Autodesk Inventor part; units mm, degrees
ref_plane "YZ Plane" through (0, 0, 0) normal (1, 0, 0) x (0, 1, 0)
ref_plane "XZ Plane" through (0, 0, 0) normal (0, 1, 0) x (-1, 0, 0)
ref_plane "XY Plane" through (0, 0, 0) normal (0, 0, 1) x (1, 0, 0)
sketch "Sketch11" plane through (0, 0, 0) normal (0, 1, 0) x (-1, 0, 0)
  circle A0 centre (0, 0) radius 26
  circle A1 centre (0, 0) radius 24
  circle A2 centre (0, 0) radius 31
  circle A3 centre (0, 0) radius 55
  line L0 (35.5726, 38.3198) -> (39.3254, 31.8198)
  line L1 (39.3254, 31.8198) -> (35.5726, 25.3198)
  line L2 (35.5726, 25.3198) -> (28.067, 25.3198)
  line L3 (28.067, 25.3198) -> (24.3143, 31.8198)
  line L4 (24.3143, 31.8198) -> (28.067, 38.3198)
  line L5 (28.067, 38.3198) -> (35.5726, 38.3198)
  line L6 (0, 0) -> (31.8198, 31.8198) construction
  line L7 (0, 0) -> (45, 0) construction
  line L8 (35.5726, 38.3198) -> (28.067, 25.3198) construction
  line L9 (28.067, 38.3198) -> (35.5726, 25.3198) construction
  line L10 (39.3254, 31.8198) -> (24.3143, 31.8198) construction
  line L11 (0, 52.6213) -> (0, 85)
  line L12 (0, 85) -> (-16, 85)
  line L13 (-16, 85) -> (-16, 52.6213)
  line L14 (0, 64) -> (0, 58.5)
  line L15 (-16, 52.6213) -> (0, 52.6213)
  line L16 (0, 52.6213) -> (-16, 52.6213)
  line L17 (-16, 52.6213) -> (-16, 44.6213)
  line L18 (-16, 44.6213) -> (0, 44.6213)
  line L19 (0, 44.6213) -> (0, 52.6213)
  line L20 (0, 68.8106) -> (-43, 68.8106)
  line L21 (-43, 68.8106) -> (-43, 250.8106)
  line L22 (-43, 250.8106) -> (0, 250.8106)
  line L23 (0, 250.8106) -> (0, 68.8106)
  dimension "oOuterDia" = 110
  dimension "oPipeDia" = 52
  dimension "oPipeWall" = 2
  dimension "oPipeLenght" = 5
  dimension "oKdia" = 45
  dimension "d70" = 45
  dimension "oSW" = 13
  dimension "oCenterTop" = 85
  dimension "d78" = 16
  dimension "d86" = 8
  dimension "oActuatorDia" = 43
  dimension "oActuatorLenght" = 182
extrude "Extrusion12" add sketch "Sketch11" along normal mid plane 52 contours A0
extrude "Extrusion13" add sketch "Sketch11" along normal mid plane 42 contours A2
extrude "Extrusion14" add sketch "Sketch11" along normal mid plane 22 contours L17 L18 L19 L11 A3 | A3 L11 L15 | L15 L19 L18 L17 | L0 L1 L2 L3 L4 L5
extrude "Extrusion15" add sketch "Sketch11" along normal mid plane 38 contours L0 L1 L2 L3 L4 L5
pattern_circular "Circular Pattern2" count 4 over 360 about axis through (0, 0, 0) along (0, 1, 0) of "Extrusion15"
revolve "Revolution1" add sketch "Sketch11" angle 360 about axis through (0, 0, 52.6213) along (0, 0, 1) contours L13 L20 L11 A3 | A3 L11 L15 | L15 L19 L18 L17 | L13 L12 L11 L20
revolve "Revolution4" add sketch "Sketch11" angle 360 about axis through (0, 0, 250.8106) along (0, 0, -1) contours L20 L21 L22 L23 L12 L13 | L13 L12 L11 L20
equation "\"d65\" = -2 * oPipeLenght + oValveLenght"
properties part number "MANUAL SANITARY BUTTERFLY VALVE 304L DN50" material "304L"
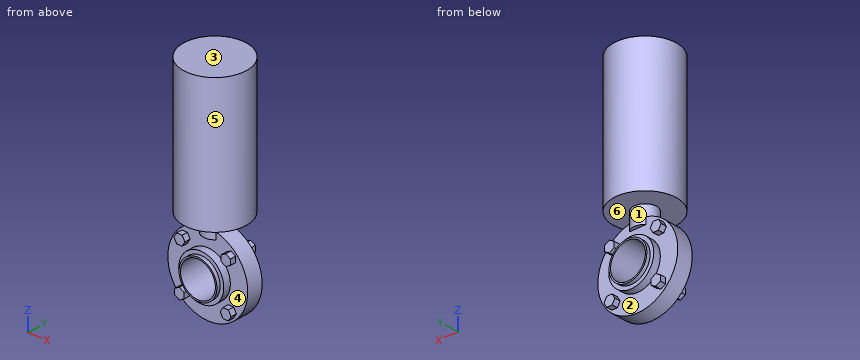
Design review of the part built by this model. Coordinates are the model's own, in mm. Face numbers are marked on the shaded views. A direction names the side the tool comes from. Round coordinates to 2 decimals unless told otherwise and drop trailing zeros. Write each loop counter-clockwise with the first axis right and the second up, starting at its lowest first coordinate (ties: lowest second). Pieces come first, ordered by that corner, then holes.
Item 1: For the marked faces 1, 2 and 3, list the 3-axis set-ups (+Z, -Z, +X, -X, +Y, -Y) from which the entire face can be reached by the end or side of a thin tool; tool diameter is ignored.
Item 2: Consider section D-D on x = -20. Give the boundary of the cut face in (y, z).
Item 3: Consider section B-B on z = 0. Give the boundary of the cut face in (x, y).
Item 4: For pin 1 Ø4 at (y, z) = (-15, 33.5) entering from -X; pin 2 Ø6 at (x, z) = (24.5, 12) entering from -Y; pin 3 Ø2.5 at (y, z) = (14.5, -33.5) entering from +X, all flat-tipped, find the tip position at first contact; note any pin that passes through.
Item 5: Consider section C-C on y = 0. Give the boundary of the cut face in (x, z), and give its area (3 significant figures).
Item 6: Draft analysis for pull direction X (two halves, no side actions). For the marked faces 4, 5 and 6, state which applies: released by +X, released by -X, zero draft, split by the parting line, or undercut.
Item 7: Wall thickness on L1, parallel to Z at x = 0, y = 12; L2, parallel to Y at x = -34, z = 13; L3, parallel to X at y = -17.5, z = 145: over which ranges is each line inside the solid? List them lowest first.
Check values:
1. face 1: none
1. face 2: +Y
1. face 3: +Z, +X, -X, +Y, -Y
2. outline: (-38.07, 68.81) - (38.07, 68.81) - (38.07, 250.81) - (-38.07, 250.81) - close; (-26, -16.61) - (-21, -16.61) - (-21, -23.69) - (-11, -23.69) - (-11, -51.23) - (11, -51.23) - (11, -23.69) - (21, -23.69) - (21, -16.61) - (26, -16.61) - (26, -13.27) - (-26, -13.27) - close; (-26, 13.27) - (26, 13.27) - (26, 16.61) - (21, 16.61) - (21, 23.69) - (11, 23.69) - (11, 51.23) - (-11, 51.23) - (-11, 23.69) - (-21, 23.69) - (-21, 16.61) - (-26, 16.61) - close
3. outline: (-55, -11) - (-31, -11) - (-31, -21) - (-26, -21) - (-26, -26) - (-24, -26) - (-24, 26) - (-26, 26) - (-26, 21) - (-31, 21) - (-31, 11) - (-55, 11) - close; (24, -26) - (26, -26) - (26, -21) - (31, -21) - (31, -11) - (55, -11) - (55, 11) - (31, 11) - (31, 21) - (26, 21) - (26, 26) - (24, 26) - close
4. pin 1: stops at x = -39.33
4. pin 2: stops at y = -26
4. pin 3: stops at x = 39.08
5. outline: (-43, 68.81) - (-16, 68.81) - (-16, 52.62) arc R55 ccw (long way) to (16, 52.62) - (16, 68.81) - (43, 68.81) - (43, 250.81) - (-43, 250.81) - close; hole circle Ø48 at (0, 0)
5. area: 23,800 mm2
6. face 4: undercut
6. face 5: split by the parting line
6. face 6: zero draft
7. L1: z = -31 to -24, 24 to 31, 44.62 to 250.81
7. L2: y = -11 to 11
7. L3: x = -39.28 to 39.28
